Autodesk Inventor part; units mm, degrees
ref_plane "YZ Plane" through (0, 0, 0) normal (1, 0, 0) x (0, 1, 0)
ref_plane "XZ Plane" through (0, 0, 0) normal (0, 1, 0) x (-1, 0, 0)
ref_plane "XY Plane" through (0, 0, 0) normal (0, 0, 1) x (1, 0, 0)
sketch "Sketch1" plane through (0, 0, 0) normal (0, 0, 1) x (1, 0, 0)
  circle A0 centre (0, 0) radius 14.8
  line L0 (-9, 21.5) -> (9, 21.5)
  line L1 (-9, 21.5) -> (-19, 11.5)
  line L2 (-19, 11.5) -> (-19, -34.776357)
  circle A1 centre (0, -34.5) radius 19
  line L3 (0, 21.5) -> (0, -34.5) construction
  line L4 (9, 21.5) -> (19, 11.5)
  line L5 (19, 11.5) -> (19, -34.776357)
  point P0 (-19, -34.5)
  point P1 (19, -34.5)
  dimension "d0" = 29.6
  dimension "d1" = 18
  dimension "d2" = 21.5
  dimension "d3" = 38
  dimension "d4" = 56
  dimension "d5" = 45
sketch "Sketch1 outline for Extrusion1" plane through (0, 0, 0) normal (0, 0, 1) x (1, 0, 0)
  line L0 (19, 11.5) -> (9, 21.5)
  line L1 (19, -34.5) -> (19, 11.5)
  arc A0 (-19, -34.5) -> (19, -34.5) centre (0, -34.5) ccw
  line L2 (-19, 11.5) -> (-19, -34.5)
  line L3 (-9, 21.5) -> (-19, 11.5)
  line L4 (9, 21.5) -> (-9, 21.5)
extrude "Extrusion1" add sketch "Sketch1 outline for Extrusion1" along normal blind 21
sketch "Sketch2" plane through (0, 0, 21) normal (0, 0, 1) x (1, 0, 0)
  line L0 (9, 21.5) -> (-9, 21.5)
  circle A0 centre (0, 0) radius 14.8
  line L1 (-9, 21.5) -> (-14.175455, 4.253996)
  line L2 (9, 21.5) -> (14.175455, 4.253996)
  line L3 (9, 21.5) -> (-9, 21.5)
  line L4 (-9, 21.5) -> (9, 21.5)
  dimension "d8" = 29.6
extrude "Extrusion2" add sketch "Sketch2" along normal blind 462.5
sketch "Sketch3" plane through (0, 0, 21) normal (0, 0, 1) x (1, 0, 0)
  arc A0 (-19, -34.5) -> (19, -34.5) centre (0, -34.5) ccw
  circle A1 centre (0, -34.5) radius 19
  point P0 (0, 0)
  point P1 (19, -34.5)
  point P2 (-19, -34.5)
extrude "Extrusion3" add sketch "Sketch3" along normal blind 74
sketch "Sketch4" plane through (-9, 21.5, 0) normal (0, 1, 0) x (1, 0, 0)
  line L0 (18, 0) -> (0, 0)
  line L1 (0, 0) -> (0, -21)
  line L2 (0, -21) -> (0, -483.5)
  line L3 (18, -483.5) -> (0, -483.5)
  line L4 (18, -21) -> (18, -483.5)
  line L5 (18, 0) -> (18, -21)
  line L6 (-16, -473) -> (34, -473)
  point P0 (9, 0)
  point P1 (9, -473)
  point P2 (9, -483.5)
  dimension "d13" = 50
  dimension "d14" = 10.5
split_face "Split1"
sketch "Sketch5" plane through (0, 0, 483.5) normal (0, 0, 1) x (1, 0, 0)
  circle A0 centre (0, 0) radius 10
  dimension "d15" = 20
extrude "Extrusion4" cut sketch "Sketch5" against normal blind 427
sketch "Sketch6" plane through (-9, 21.5, 0) normal (0, 1, 0) x (1, 0, 0)
  line L0 (18, -473) -> (0, -473)
  line L1 (18, -21) -> (18, -473)
  line L2 (18, 0) -> (18, -21)
  line L3 (18, 0) -> (0, 0)
  line L4 (0, 0) -> (0, -21)
  line L5 (0, -21) -> (0, -473)
  line L6 (18, -473) -> (0, -473)
  line L7 (0, -473) -> (0, -483.5)
  line L8 (18, -483.5) -> (0, -483.5)
  line L9 (18, -473) -> (18, -483.5)
  point P0 (9, 0)
  point P1 (9, -467.5)
  point P2 (9, -28)
  point P3 (9, 0)
  point P4 (9, -483.5)
  dimension "d18" = 28
  dimension "d19" = 16
hole "Hole1" at (0, 21.5, 467.5) at (0, 21.5, 28) direction (0, -1, 0) diameter 3.242 depth 8 countersink diameter 7 countersink angle 90
properties part number "Linear Motor (T-Frame)" material "Aluminum 6061"
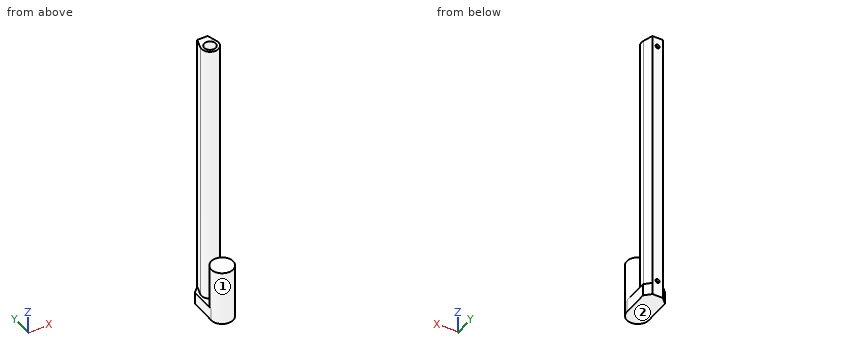
Input: part model. Units: mm. Frame: model coordinates. Face numbers are marked on the shaded views. Round coordinates to 2 decimals unless told otherwise and drop trailing zeros. Write each loop counter-clockwise with the first axis right and the second up, starting at its lowest first coordinate (ties: lowest second). Pieces come first, ordered by that corner, then holes.
1) Contact query for flat-ended pins moving along their axis: P1, Ø2.5, axis at x = 0, z = 28, coming from the -Y side; P2, Ø3, axis at x = 0, z = 467.5, coming from the -Y side; P3, Ø4, axis at x = -0.5, y = -40.5, coming from the +Z side; P4, Ø22, axis at x = 2.5, y = 4, coming from the +Z side. Output: stop coordinate, or through.
2) Cut plane C-C (y = -27). Return the cut outline in (x, z), then the cut area to 3 significant figures.
3) Ray query, L1, parallel to Z at x = 0, y = 15.75; L2, parallel to Y at x = 0, z = 233; L3, parallel to Y at x = -7, z = 66. Return the intervals inside material, ascending.
4) Cut plane B-B (z = 246). Return the cut outline in (x, y).
5) Draft query along Y for the marked faces 1 and 2. Return one class per face: pulls with the +Y half, pulls with the -Y half, needs draft (parallel to the pull), parting line crosses it, or undercut.
6) Cut plane A-A (y = 0). Return the cut outline in (x, z), then the cut area to 3 significant figures.
Geometry says:
1. P1: stops at y = -53.5
1. P2: stops at y = -14.8
1. P3: stops at z = 95
1. P4: stops at z = 483.5
2. outline: (-19, 0) - (19, 0) - (19, 21) - (17.46, 21) - (17.46, 95) - (-17.46, 95) - (-17.46, 21) - (-19, 21) - close
2. area: 3,380 mm2
3. L1: z = 0 to 26.38, 29.62 to 465.88, 469.12 to 483.5
3. L2: y = -14.8 to -10, 10 to 21.5
3. L3: y = -52.16 to -16.84, -13.04 to -7.14, 7.14 to 21.5
4. outline: (-14.18, 4.25) arc R14.8 ccw (long way) to (14.18, 4.25) - (9, 21.5) - (-9, 21.5) - close; hole circle Ø20 at (0, 0)
5. face 1: undercut
5. face 2: needs draft
6. outline: (-19, 0) - (19, 0) - (19, 21) - (14.8, 21) - (14.8, 483.5) - (10, 483.5) - (10, 56.5) - (-10, 56.5) - (-10, 483.5) - (-14.8, 483.5) - (-14.8, 21) - (-19, 21) - close
6. area: 5,950 mm2
